The listing builds one solid part. Answer for the finished solid, in the listing's coordinates (mm). Face numbers are marked on the shaded views. A direction names the side the tool comes from. Give positions to 0.01 mm unless a question says otherwise; leave off trailing zeros. Loops run counter-clockwise (first coordinate to the right, second up) from the corner with the lowest first, then second, coordinate; pieces in that order, holes last. Notation, with made-up numbers: (-5, -18.75) - (50, -18.75) arc R17 cw to (50, -2.75) - close; hole circle Ø6 at (-3.5, 40.25). An arc over 180 degrees is marked (long way). Answer as CSV lines item,"result". Start each with the question number.
1) A cutting plane is placed at A-A (x = -54). Determine the outline of the cut face in (y, z).
2) A cutting plane is placed at B-B (z = 70). Give the number of separate pieces and of enclosed holes in the cut face, and give its area (3 significant figures).
3) For the marked faces 1, 2 and 3, determine the directions among +Z, -Z, +X, -X, +Y, -Y from which every point of the face is accessible in a straight line to the end or side of a thin tool.
4) Flat-ended cylindrical pins translate along their axes: pin 1 (16 mm diameter, centred on x = -54, y = 19.5, fed in from -Z); pin 2 (2 mm diameter, centred on x = -8.5, z = 39, fed in from +Y); pin 3 (11.5 mm diameter, centred on x = 22.5, z = 70, fed in from -Y); pin 4 (5 mm diameter, centred on x = 51, z = 41.5, fed in from -Y). Find the tip coordinate at first contact, or state that the pin passes through.
5) A cutting plane is placed at C-C (x = -30). Determine the outline of the cut face in (y, z), and give its area (3 significant figures).
6) Find the intervals of material crossed by line 1 along Y through (x, z) = (54, 46.5); line 2 along X through (y, z) = (-19, 50); line 3 along X through (y, z) = (3, 13), in increasing order.
7) A cutting plane is placed at D-D (z = 56). Determine the outline of the cut face in (x, y), and give its area (3 significant figures).
8) For a pull along X with two mould halves and no side action, classify the marked faces 4, 5 and 6 as pulls with the +X half, pulls with the -X half, needs draft (parallel to the pull), parting line crosses it, or undercut.
```python
from build123d import *

# Parameters (mm, degrees)
F1_DEPTH = 80
F2_R     = 5
F3_DEPTH = 25


with BuildPart() as f1:
    # F0 (on Top) → F1 (new body)
    with BuildSketch(Plane.XY):
        with BuildLine():
            Line((44, 7), (63, 7))
            ThreePointArc((63, 7), (63.707107, 6.707107), (64, 6))
            Line((64, 6), (64, -6))
            ThreePointArc((64, -6), (63.707107, -6.707107), (63, -7))
            Line((63, -7), (44, -7))
            Line((44, -7), (44, -19.5))
            ThreePointArc((44, -19.5), (54, -9.5), (64, -19.5))
            Line((64, -19.5), (64, -7))
            Line((64, -7), (66, -7))
            Line((66, -7), (66, 7))
            Line((66, 7), (64, 7))
            Line((64, 7), (64, 19.5))
            ThreePointArc((64, 19.5), (54, 9.5), (44, 19.5))
            Line((44, 19.5), (44, 7))
        make_face()
        with BuildLine():
            Line((42, 7), (44, 7))
            Line((44, 7), (44, 19.5))
            ThreePointArc((44, 19.5), (54, 29.5), (64, 19.5))
            Line((64, 19.5), (64, 7))
            Line((64, 7), (66, 7))
            Line((66, 7), (66, 19.5))
            ThreePointArc((66, 19.5), (54, 31.5), (42, 19.5))
            Line((42, 19.5), (42, 7))
        make_face()
        with BuildLine():
            Line((-42, 7), (42, 7))
            Line((42, 7), (42, 19.5))
            ThreePointArc((42, 19.5), (39.071068, 12.428932), (32, 9.5))
            Line((32, 9.5), (-32, 9.5))
            ThreePointArc((-32, 9.5), (-39.071068, 12.428932), (-42, 19.5))
            Line((-42, 19.5), (-42, 7))
        make_face()
        with BuildLine():
            Line((-44, 7), (-42, 7))
            Line((-42, 7), (-42, 19.5))
            ThreePointArc((-42, 19.5), (-54, 31.5), (-66, 19.5))
            Line((-66, 19.5), (-66, 7))
            Line((-66, 7), (-64, 7))
            Line((-64, 7), (-64, 19.5))
            ThreePointArc((-64, 19.5), (-54, 29.5), (-44, 19.5))
            Line((-44, 19.5), (-44, 7))
        make_face()
        with BuildLine():
            Line((-63, 7), (-44, 7))
            Line((-44, 7), (-44, 19.5))
            ThreePointArc((-44, 19.5), (-54, 9.5), (-64, 19.5))
            Line((-64, 19.5), (-64, 7))
            Line((-64, 7), (-66, 7))
            Line((-66, 7), (-66, -6.902831))
            Line((-66, -6.902831), (-64, -7))
            Line((-64, -7), (-64, -19.5))
            ThreePointArc((-64, -19.5), (-54, -9.5), (-44, -19.5))
            Line((-44, -19.5), (-44, -7))
            Line((-44, -7), (-63, -7))
            ThreePointArc((-63, -7), (-63.707107, -6.707107), (-64, -6))
            Line((-64, -6), (-64, 6))
            ThreePointArc((-64, 6), (-63.707107, 6.707107), (-63, 7))
        make_face()
        with BuildLine():
            Line((44, -19.5), (44, -7))
            Line((44, -7), (42, -7))
            Line((42, -7), (42, -19.5))
            ThreePointArc((42, -19.5), (54, -31.5), (66, -19.5))
            Line((66, -19.5), (66, -7))
            Line((66, -7), (64, -7))
            Line((64, -7), (64, -19.5))
            ThreePointArc((64, -19.5), (54, -29.5), (44, -19.5))
        make_face()
        with BuildLine():
            Line((42, -19.5), (42, -7))
            Line((42, -7), (-42, -7))
            Line((-42, -7), (-42, -19.5))
            ThreePointArc((-42, -19.5), (-39.071068, -12.428932), (-32, -9.5))
            Line((-32, -9.5), (32, -9.5))
            ThreePointArc((32, -9.5), (39.071068, -12.428932), (42, -19.5))
        make_face()
        with BuildLine():
            Line((-42, -19.5), (-42, -7))
            Line((-42, -7), (-44, -7))
            Line((-44, -7), (-44, -19.5))
            ThreePointArc((-44, -19.5), (-54, -29.5), (-64, -19.5))
            Line((-64, -19.5), (-64, -7))
            Line((-64, -7), (-66, -6.902831))
            Line((-66, -6.902831), (-66, -19.5))
            ThreePointArc((-66, -19.5), (-54, -31.5), (-42, -19.5))
        make_face()
    extrude(amount=F1_DEPTH)

    # F2 (on Front) → F3 (cut)
    with BuildSketch(Plane.XZ):
        with Locations((22.5, 70)):
            Circle(F2_R)
        with Locations((7.5, 70)):
            Circle(F2_R)
    extrude(amount=-F3_DEPTH, mode=Mode.SUBTRACT)


solid = f1.part
```
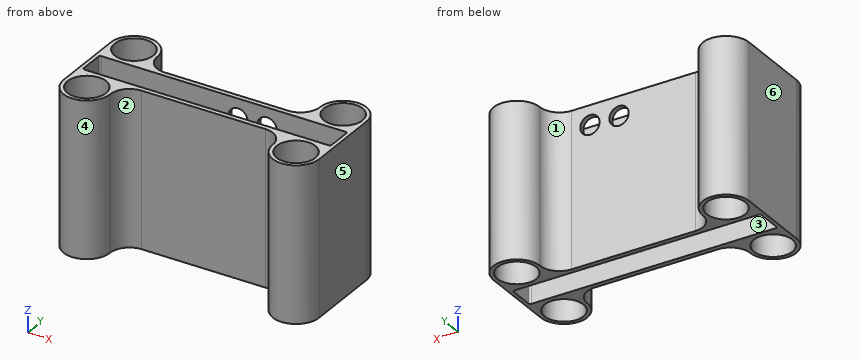
Ans:
1,outline,"(-31.5, 0) - (-29.5, 0) - (-29.5, 80) - (-31.5, 80) - close; (-9.5, 0) - (-7, 0) - (-7, 80) - (-9.5, 80) - close; (7, 0) - (9.5, 0) - (9.5, 80) - (7, 80) - close; (29.5, 0) - (31.5, 0) - (31.5, 80) - (29.5, 80) - close"
2,separate pieces,"2"
2,enclosed holes,"4"
2,area,"1,360 mm2"
3,face 1,"+Z, -Z, +Y"
3,face 2,"+Z, -Z, -Y"
3,face 3,"+Z, -Z"
4,pin 1,"through"
4,pin 2,"y = 9.5"
4,pin 3,"y = -9.5"
4,pin 4,"y = -31.49"
5,outline,"(-9.5, 0) - (-7, 0) - (-7, 80) - (-9.5, 80) - close; (7, 0) - (9.5, 0) - (9.5, 80) - (7, 80) - close"
5,area,"400 mm2"
6,line 1,"-31.5 to -29.5, -9.5 to -7, 7 to 9.5, 29.5 to 31.5"
6,line 2,"-66 to -63.99, -44.01 to -41.99, 41.99 to 44.01, 63.99 to 66"
6,line 3,"-66 to -64, 64 to 66"
7,outline,"(-66, -19.5) arc R12 ccw to (-42, -19.5) arc R10 cw to (-32, -9.5) - (32, -9.5) arc R10 cw to (42, -19.5) arc R12 ccw to (66, -19.5) - (66, 19.5) arc R12 ccw to (42, 19.5) arc R10 cw to (32, 9.5) - (-32, 9.5) arc R10 cw to (-42, 19.5) arc R12 ccw to (-66, 19.5) - close; hole circle Ø20 at (-54, -19.5); hole (-64, -6) arc R1 ccw to (-63, -7) - (63, -7) arc R1 ccw to (64, -6) - (64, 6) arc R1 ccw to (63, 7) - (-63, 7) arc R1 ccw to (-64, 6) - close; hole circle Ø20 at (-54, 19.5); hole circle Ø20 at (54, -19.5); hole circle Ø20 at (54, 19.5)"
7,area,"1,410 mm2"
8,face 4,"undercut"
8,face 5,"pulls with the +X half"
8,face 6,"pulls with the -X half"
